Design review of the part shown in the three views and the two pictorial views. Dimensions are in mm from the part's minimum x, y and z. Round coordinates to 2 decimals unless told otherwise and drop trailing zeros. Write each loop counter-clockwise with the first axis right and the second up, starting at its lowest first coordinate (ties: lowest second). Pieces come first, ordered by that corner, then holes. Notation, with made-up numbers: (-24.75, 31) - (-19.75, 31) arc R16 ccw to (-19.75, 37) - close; hole circle Ø10 at (25.25, 71). An arc over 180 degrees is marked (long way). Use one line per item in the form item = value.
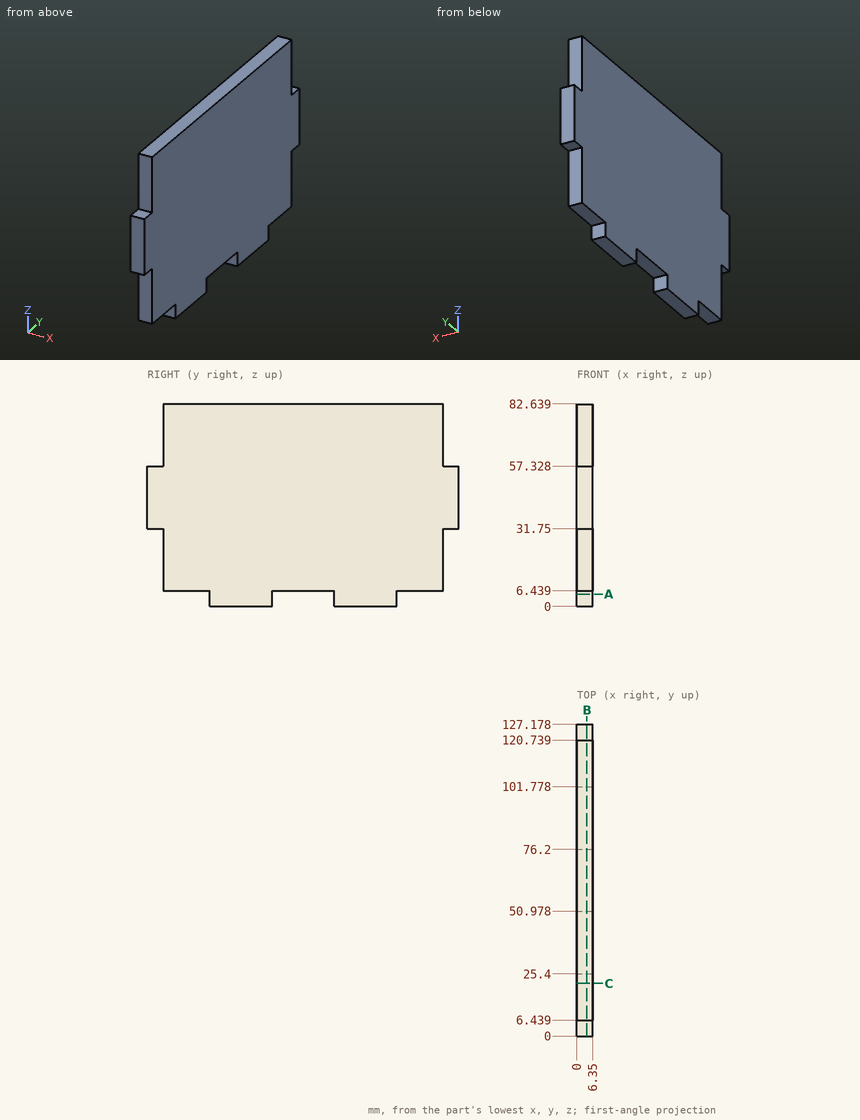
Q1. We need section A-A on z = 5. Write out the cut boundary in (x, y), then the cut area to 3 significant figures.
Calculated:
outline = (0, 25.4) - (6.35, 25.4) - (6.35, 50.98) - (0, 50.98) - close; (0, 76.2) - (6.35, 76.2) - (6.35, 101.78) - (0, 101.78) - close
area = 325 mm2
Q2. For P1, Ø1.9, axis at x = 3.5, y = 124, coming from the +Z side; P2, Ø1.9, axis at x = 3, z = 15.5, coming from the +Y side; P3, Ø1.9, axis at x = 2, y = 122.5, coming from the -Z side, all flat-tipped, find the tip position at first contact; note any pin that passes through.
Calculated:
P1 = 57.33
P2 = 120.74
P3 = 31.75
Q3. To check wall thickness, follow line 1 along Y through (x, z) = (3.5, 4); line 2 along Z through (x, y) = (4.5, 52); line 3 along Y through (x, z) = (1.5, 23). State the ranges of each line that lie inside material, in increasing order. Write a range as from..to.
Calculated:
line_1 = 25.4..50.98, 76.2..101.78
line_2 = 6.44..82.64
line_3 = 6.44..120.74
Q4. We need section B-B on x = 4. Write out the cut boundary in (y, z).
Calculated:
outline = (0, 31.75) - (6.44, 31.75) - (6.44, 6.44) - (25.4, 6.44) - (25.4, 0) - (50.98, 0) - (50.98, 6.44) - (76.2, 6.44) - (76.2, 0) - (101.78, 0) - (101.78, 6.44) - (120.74, 6.44) - (120.74, 31.75) - (127.18, 31.75) - (127.18, 57.33) - (120.74, 57.33) - (120.74, 82.64) - (6.44, 82.64) - (6.44, 57.33) - (0, 57.33) - close
Q5. We need section C-C on y = 21.5. Write out the cut boundary in (x, z), then the cut area to 3 significant figures.
Calculated:
outline = (0, 6.44) - (6.35, 6.44) - (6.35, 82.64) - (0, 82.64) - close
area = 484 mm2
